```python
from build123d import *

# Parameters (mm, degrees)
SKETCH1_R                = 8
BOSS_EXTRUDE1_DEPTH      = 2
SKETCH2_R                = 9
BOSS_EXTRUDE2_DEPTH      = 3
CUT_EXTRUDE1_DEPTH       = 10.0001
CUT_EXTRUDE1_DEPTH_BACK  = 10
BOSS_EXTRUDE3_DEPTH      = 2
BOSS_EXTRUDE3_DEPTH_BACK = 0.0001
SKETCH1_3_R              = 8
SKETCH3_R                = 4
BOSS_EXTRUDE4_DEPTH      = 20


with BuildPart() as part:
    # Sketch1 → Boss-Extrude1 (new body)
    with BuildSketch(Plane.XY):
        Circle(SKETCH1_R)
        with BuildLine():
            Line((-2.100590034, 1.75), (2.142050653, 1.75))
            ThreePointArc((2.142050653, 1.75), (2.766022596, 0), (2.142050653, -1.75))
            Line((2.142050653, -1.75), (-2.100590034, -1.75))
            ThreePointArc((-2.100590034, -1.75), (-2.733195007, 0), (-2.100590034, 1.75))
        make_face(mode=Mode.SUBTRACT)
    extrude(amount=BOSS_EXTRUDE1_DEPTH)

    # Sketch2 → Boss-Extrude2 (add)
    with BuildSketch(Plane.XY.offset(2)):
        Circle(SKETCH2_R)
    extrude(amount=-BOSS_EXTRUDE2_DEPTH)

    # Sketch1_2 → Cut-Extrude1 (cut, two sides: drawn at the far end of the back side and taken through both)
    with BuildSketch(Plane.XY.offset(-CUT_EXTRUDE1_DEPTH_BACK)):
        with BuildLine():
            ThreePointArc((-2.100590034, -1.75), (-2.733195007, 0), (-2.100590034, 1.75))
            Line((-2.100590034, 1.75), (2.142050653, 1.75))
            ThreePointArc((2.142050653, 1.75), (2.766022596, 0), (2.142050653, -1.75))
            Line((2.142050653, -1.75), (-2.100590034, -1.75))
        make_face()
    extrude(amount=CUT_EXTRUDE1_DEPTH + CUT_EXTRUDE1_DEPTH_BACK, mode=Mode.SUBTRACT)

    # Sketch1_3 → Boss-Extrude3 (add, two sides: drawn at the far end of the back side and taken through both)
    with BuildSketch(Plane.XY.offset(-BOSS_EXTRUDE3_DEPTH_BACK)):
        Circle(SKETCH1_3_R)
    extrude(amount=BOSS_EXTRUDE3_DEPTH + BOSS_EXTRUDE3_DEPTH_BACK)

    # Sketch3 → Boss-Extrude4 (add)
    with BuildSketch(Plane.XY.offset(2)):
        with Locations((-0.074058603, 0.074058603)):
            Circle(SKETCH3_R)
    extrude(amount=BOSS_EXTRUDE4_DEPTH)


solid = part.part
```
Geometry: final body of the model. Coordinates: model frame, mm. A direction names the side the tool comes from. Give positions to 0.01 mm unless a question says otherwise; leave off trailing zeros. Order: outer loops, then holes, each group sorted by start corner. A loop starts at its lowest first (then second) coordinate and runs counter-clockwise, first axis right, second up. Notation, with made-up numbers: (63.25, 58.5) -> (72.25, 58.5) arc R20 cw to (72.25, 68.5) -> close; hole circle Ø5 at (2, 67.5). An arc over 180 degrees is marked (long way). Write each question's results on one line, items separated by ' | '. Start each with the question number.
1) Draft query along X for faces 4 (the flat face through (4, -2, 2)), 5 (the flat face through (0.1, -1.75, -0.5)), 6 (the flat face through (0, 1.75, -0.5)), 7 (the cylindrical face through (-1.172, 8.923, 0.521)). Return one class per face: pulls with the +X half, pulls with the -X half, needs draft (parallel to the pull), parting line crosses it, or undercut.
2) Section B-B (y = -0.75). Return loops of the section in (x, z).
3) First-contact query: pin 1 (3 mm diameter, centred on y = 3, z = 4, fed in from +X); pin 2 (0.8 mm diameter, centred on x = -1, z = -0.5, fed in from +Y); pin 3 (10 mm diameter, centred on y = -5.5, z = 13, fed in from +X). Flat tips, straight axial feed; report the tip coordinate or a pass-through.
4) Section C-C (z = 18.75). Return loops of the section in (x, y), then the cut area to 3 significant figures.
5) Line query: line 1 (Z direction, x = 0.25, y = -1.5); line 2 (Z direction, x = 4, y = 3.75); line 3 (X direction, y = -3.25, z = 7.25). Output: solid intervals per line, ascending. Write a range as from..to.
6) Set-up query: faces 1 (the cylindrical face through (2.766, 0.027, -0.507)), 2 (the cylindrical face through (-0.94, -3.83, 11.86)), 3 (the flat face through (0, 0, 22)). Return all of +Z, -Z, +X, -X, +Y, -Y with unobstructed straight access to the full face (end or side cutting, diameter ignored); none if empty.
7) Section A-A (x = 0). Return loops of the section in (y, z).
8) Section D-D (x = 5.5). Return loops of the section in (y, z), then the cut area to 3 significant figures.
Calculated:
1) face 4: needs draft | face 5: undercut | face 6: undercut | face 7: parting line crosses it
2) outline: (-8.97, -1) -> (-2.63, -1) -> (-2.63, 0) -> (2.66, 0) -> (2.66, -1) -> (8.97, -1) -> (8.97, 2) -> (3.84, 2) -> (3.84, 22) -> (-3.99, 22) -> (-3.99, 2) -> (-8.97, 2) -> close
3) pin 1: x = 3.66 | pin 2: y = 8.98 | pin 3: x = 3.88
4) outline: circle Ø8 at (-0.07, 0.07) | area: 50.3 mm2
5) line 1: 0..22 | line 2: -1..2 | line 3: -2.3..2.15
6) face 1: -Z | face 2: +Z | face 3: +Z, +X, -X, +Y, -Y
7) outline: (-9, -1) -> (-1.75, -1) -> (-1.75, 0) -> (1.75, 0) -> (1.75, -1) -> (9, -1) -> (9, 2) -> (4.07, 2) -> (4.07, 22) -> (-3.93, 22) -> (-3.93, 2) -> (-9, 2) -> close
8) outline: (-7.12, -1) -> (7.12, -1) -> (7.12, 2) -> (-7.12, 2) -> close | area: 42.7 mm2
